Read the model definition and answer for the solid it produces. Units are mm, in the model's axes. Face numbers are marked on the shaded views. A direction names the side the tool comes from. Give positions to 0.01 mm unless a question says otherwise; leave off trailing zeros. Order: outer loops, then holes, each group sorted by start corner. A loop starts at its lowest first (then second) coordinate and runs counter-clockwise, first axis right, second up. Notation, with made-up numbers: M -5.75,-39 L 29.25,-39 A20 ccw 29.25,-20 Z; hole C 89,15.25 d1. An arc over 180 degrees is marked long. One line per item, written item: value.
from build123d import *

# Parameters (mm, degrees)
SKETCH1_W           = 72.5
SKETCH1_H           = 39.8
BOSS_EXTRUDE1_DEPTH = 2.85
BOSS_EXTRUDE2_DEPTH = 23.1
SKETCH5_W           = 42.2
SKETCH5_H           = 42.1
CUT_EXTRUDE1_DEPTH  = 37.8
CUT_EXTRUDE2_REACH  = 71.017
SKETCH6_R           = 1.45
SKETCH6_R_2         = 11.9
FILLET1_R           = 3
BOSS_EXTRUDE3_DEPTH = 1


with BuildPart() as part:
    # Sketch1 → Boss-Extrude1 (new body)
    with BuildSketch(Plane.XY):
        Rectangle(SKETCH1_W, SKETCH1_H)
        with BuildLine():
            Line((-27.9, 10.05), (-27.9, 7.45))
            ThreePointArc((-27.9, 7.45), (-30, 5.35), (-32.1, 7.45))
            Line((-32.1, 7.45), (-32.1, 10.05))
            ThreePointArc((-32.1, 10.05), (-30, 12.15), (-27.9, 10.05))
        make_face(mode=Mode.SUBTRACT)
        with BuildLine():
            Line((-27.9, -10.05), (-27.9, -7.45))
            ThreePointArc((-27.9, -7.45), (-30, -5.35), (-32.1, -7.45))
            Line((-32.1, -7.45), (-32.1, -10.05))
            ThreePointArc((-32.1, -10.05), (-30, -12.15), (-27.9, -10.05))
        make_face(mode=Mode.SUBTRACT)
        with BuildLine():
            Line((27.9, 10.05), (27.9, 7.45))
            ThreePointArc((27.9, 7.45), (30, 5.35), (32.1, 7.45))
            Line((32.1, 7.45), (32.1, 10.05))
            ThreePointArc((32.1, 10.05), (30, 12.15), (27.9, 10.05))
        make_face(mode=Mode.SUBTRACT)
        with BuildLine():
            Line((27.9, -10.05), (27.9, -7.45))
            ThreePointArc((27.9, -7.45), (30, -5.35), (32.1, -7.45))
            Line((32.1, -7.45), (32.1, -10.05))
            ThreePointArc((32.1, -10.05), (30, -12.15), (27.9, -10.05))
        make_face(mode=Mode.SUBTRACT)
    extrude(amount=BOSS_EXTRUDE1_DEPTH)

    # Sketch4 → Boss-Extrude2 (add, symmetric)
    with BuildSketch(Plane(origin=(0, 0, 0), x_dir=(0, 0, -1), z_dir=(1, 0, 0))):
        Polygon((-2.85, 19.1), (-44.95, -17.9), (-44.95, -19.9), (-2.85, -19.9), align=None)
    extrude(amount=BOSS_EXTRUDE2_DEPTH, both=True)

    # Sketch5 → Cut-Extrude1 (cut)
    with BuildSketch(Plane(origin=(0, 19.9, 0), x_dir=(1, 0, 0), z_dir=(0, 1, 0))):
        with Locations((0, -23.9)):
            Rectangle(SKETCH5_W, SKETCH5_H)
    extrude(amount=-CUT_EXTRUDE1_DEPTH, mode=Mode.SUBTRACT)

    # Sketch6 → Cut-Extrude2 (cut, up to next)
    with BuildSketch(Plane(origin=(0, -17.9, 0), x_dir=(1, 0, 0), z_dir=(0, 1, 0)), mode=Mode.PRIVATE) as cut_extrude2_sk1:
        with Locations(Location((-15.5, -8, 0), (0, 0, 270))):
            Circle(SKETCH6_R)
    cut_extrude2_tool1 = extrude(cut_extrude2_sk1.sketch, amount=-CUT_EXTRUDE2_REACH, mode=Mode.PRIVATE) & part.part
    # Sketch6 → Cut-Extrude2 (cut, up to next)
    with BuildSketch(Plane(origin=(0, -17.9, 0), x_dir=(1, 0, 0), z_dir=(0, 1, 0)), mode=Mode.PRIVATE) as cut_extrude2_sk2:
        with Locations(Location((15.5, -8, 0), (0, 0, 270))):
            Circle(SKETCH6_R)
    cut_extrude2_tool2 = extrude(cut_extrude2_sk2.sketch, amount=-CUT_EXTRUDE2_REACH, mode=Mode.PRIVATE) & part.part
    # Sketch6 → Cut-Extrude2 (cut, up to next)
    with BuildSketch(Plane(origin=(0, -17.9, 0), x_dir=(1, 0, 0), z_dir=(0, 1, 0)), mode=Mode.PRIVATE) as cut_extrude2_sk3:
        with Locations(Location((15.5, -39, 0), (0, 0, 270))):
            Circle(SKETCH6_R)
    cut_extrude2_tool3 = extrude(cut_extrude2_sk3.sketch, amount=-CUT_EXTRUDE2_REACH, mode=Mode.PRIVATE) & part.part
    # Sketch6 → Cut-Extrude2 (cut, up to next)
    with BuildSketch(Plane(origin=(0, -17.9, 0), x_dir=(1, 0, 0), z_dir=(0, 1, 0)), mode=Mode.PRIVATE) as cut_extrude2_sk4:
        with Locations(Location((-15.5, -39, 0), (0, 0, 270))):
            Circle(SKETCH6_R)
    cut_extrude2_tool4 = extrude(cut_extrude2_sk4.sketch, amount=-CUT_EXTRUDE2_REACH, mode=Mode.PRIVATE) & part.part
    # Sketch6 → Cut-Extrude2 (cut, up to next)
    with BuildSketch(Plane(origin=(0, -17.9, 0), x_dir=(1, 0, 0), z_dir=(0, 1, 0)), mode=Mode.PRIVATE) as cut_extrude2_sk5:
        with Locations(Location((0, -23.5, 0), (0, 0, 270))):
            Circle(SKETCH6_R_2)
    cut_extrude2_tool5 = extrude(cut_extrude2_sk5.sketch, amount=-CUT_EXTRUDE2_REACH, mode=Mode.PRIVATE) & part.part
    add(cut_extrude2_tool1.solids().sort_by_distance((-15.5, -17.9, 8))[0], mode=Mode.SUBTRACT)
    add(cut_extrude2_tool2.solids().sort_by_distance((15.5, -17.9, 8))[0], mode=Mode.SUBTRACT)
    add(cut_extrude2_tool3.solids().sort_by_distance((15.5, -17.9, 39))[0], mode=Mode.SUBTRACT)
    add(cut_extrude2_tool4.solids().sort_by_distance((-15.5, -17.9, 39))[0], mode=Mode.SUBTRACT)
    add(cut_extrude2_tool5.solids().sort_by_distance((0, -17.9, 23.5))[0], mode=Mode.SUBTRACT)

    # Fillet1
    fillet1_edges = [part.edges().sort_by_distance(p)[0] for p in [
        (-36.25, 19.9, 1.425),
        (36.25, 19.9, 1.425),
        (36.25, -19.9, 1.425),
        (-36.25, -19.9, 1.425),
    ]]
    fillet(fillet1_edges, radius=FILLET1_R)

    # Sketch7 → Boss-Extrude3 (add, symmetric)
    with BuildSketch(Plane(origin=(0, 0, 0), x_dir=(1, 0, 0), z_dir=(0, 1, 0))):
        Polygon((34.25, -2.85), (23.1, -18.85), (23.1, -2.85), align=None)
        Polygon((-23.1, -2.85), (-34.25, -2.85), (-23.1, -18.85), align=None)
    extrude(amount=BOSS_EXTRUDE3_DEPTH, both=True)


solid = part.part
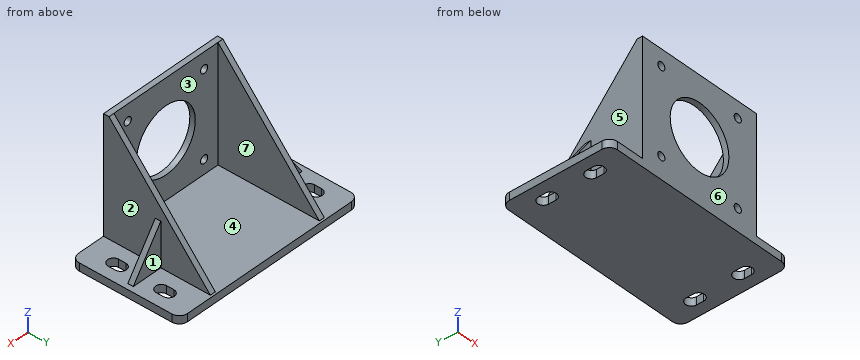
1) Find section D-D, the plane z = 39. Write down the section's boundary in (x, y).
Reported:
outline: M -23.1,-19.9 L -16.95,-19.9 L -16.95,-17.9 L -21.1,-17.9 L -21.1,-12.67 L -23.1,-12.67 Z; M -14.05,-19.9 L 14.05,-19.9 L 14.05,-17.9 L -14.05,-17.9 Z; M 16.95,-19.9 L 23.1,-19.9 L 23.1,-12.67 L 21.1,-12.67 L 21.1,-17.9 L 16.95,-17.9 Z
2) Which of the six approach directions +Z, -Z, +X, -X, +Y, -Y give full straight-line access (tool end or side, diameter ignored) to the marked faces 1, 2 and 3?
Reported:
face 1: +Z, +X, +Y
face 2: +Z, +X
face 3: +Z, +Y
3) Find section A-A, the plane z = 23.5. Write down the section's boundary in (x, y).
Reported:
outline: M -23.1,-19.9 L -11.9,-19.9 L -11.9,-17.9 L -21.1,-17.9 L -21.1,0.95 L -23.1,0.95 Z; M 11.9,-19.9 L 23.1,-19.9 L 23.1,0.95 L 21.1,0.95 L 21.1,-17.9 L 11.9,-17.9 Z
4) Consider probe 1 along X at (y, z) = (-19, 8); probe 2 along X at (y, z) = (-19, 23); probe 3 along X at (y, z) = (-9.5, 4.5). Determine where each line is inside the solid, lowest interval first.
Reported:
probe 1: x = -23.1 to -16.95, -14.05 to 14.05, 16.95 to 23.1
probe 2: x = -23.1 to -11.89, 11.89 to 23.1
probe 3: x = -23.1 to -21.1, 21.1 to 23.1
5) Find section C-C, the plane y = -15. Write down the section's boundary in (x, z), plus the area to 3 significant figures.
Reported:
outline: M -36.25,0 L 36.25,0 L 36.25,2.85 L 23.1,2.85 L 23.1,41.65 L 21.1,41.65 L 21.1,2.85 L -21.1,2.85 L -21.1,41.65 L -23.1,41.65 L -23.1,2.85 L -36.25,2.85 Z
area: 362 mm^2
6) Each of these flat-tipped pins is pushed along its axis until it touches: pin 1 Ø11.5 at (y, z) = (-10, 25.5) entering from -X; pin 2 Ø1.5 at (x, z) = (-24.5, 14.5) entering from +Y; pin 3 Ø4 at (x, z) = (0, 6) entering from +Y. Where does it stop, or does it pass through?
Reported:
pin 1: stops at x = -23.1
pin 2: stops at y = 1
pin 3: stops at y = -17.9
7) Determine the mould class of the marked faces 4, 5, 6 and 7 for opening direction X: +X half, -X half, draft (parallel to the pull), parting line (faces both ways), or undercut.
Reported:
face 4: undercut
face 5: -X half
face 6: draft
face 7: undercut
8) Find section B-B, the plane x = 30. Write down the section's boundary in (y, z).
Reported:
outline: M -19.9,0 L -12.15,0 L -12.15,2.85 L -19.9,2.85 Z; M -5.35,0 L 5.35,0 L 5.35,2.85 L 1,2.85 L 1,8.95 L -1,8.95 L -1,2.85 L -5.35,2.85 Z; M 12.15,0 L 19.9,0 L 19.9,2.85 L 12.15,2.85 Z
